Geometry: final body of the model. Coordinates: model frame, mm. Coordinates: 2 decimals unless noted, no trailing zeros. Order: outer loops, then holes, each group sorted by start corner. A loop starts at its lowest first (then second) coordinate and runs counter-clockwise, first axis right, second up. Notation, with made-up numbers: (9, -6.5) -> (28, -6.5) arc R32 ccw to (28, 24.5) -> close; hole circle Ø6 at (-38.75, 4). An arc over 180 degrees is marked (long way). Use one line per item in the form item = value.
Autodesk Fusion 360 part; units mm, degrees
sketch "Sketch1" plane through (0, 0, 0) normal (0, 0, 1) x (1, 0, 0)
  line L0 (0, 0) -> (50, 0)
  line L1 (50, 0) -> (50, 50)
  line L2 (50, 50) -> (0, 50)
  line L3 (0, 50) -> (0, 0)
  line L4 (25, 59.9444) -> (25, -10) construction
  line L5 (-9.9209, 25) -> (60, 25) construction
  line L6 (23.4218, 51.9444) -> (26.5218, 51.9444)
  line L7 (26.5218, 51.9444) -> (26.5218, 25)
  line L8 (26.5218, 25) -> (23.4218, 25)
  line L9 (23.4218, 25) -> (23.4218, 51.9444)
  dimension "d4" = 3.1
extrude "Extrude1" add sketch "Sketch1" along normal blind 3.2 contours L0 L1 L2 L3 L7 L8 L9
chamfer "Chamfer1" distance 3 angle 45 2 edges at (26.5218, 50, 1.6) (23.4218, 50, 1.6)
equation "material_thickness = 3.2 mm"
equation "laser_kerf = 0.1 mm"
equation "chamfer_amount = 3 mm"
equation "d4 = material_thickness - laser_kerf"
equation "d5 = material_thickness"
equation "d7 = chamfer_amount"
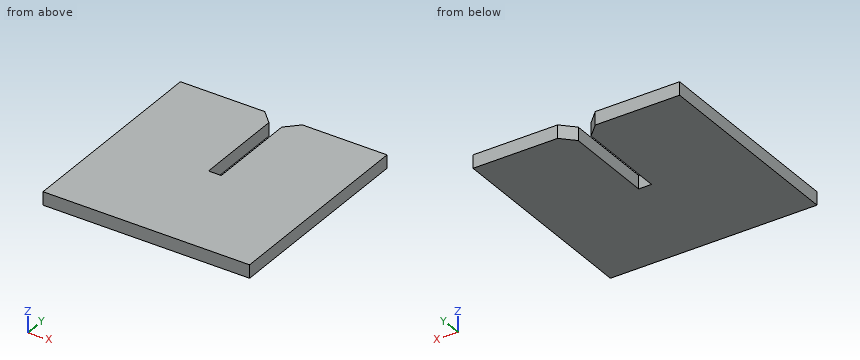
1) Contact query for flat-ended pins moving along their axis: P1, Ø4, axis at x = 16.5, y = 12.5, coming from the -Z side; P2, Ø1.5, axis at x = 25.5, z = 2.5, coming from the +Y side. Output: stop coordinate, or through.
Results found:
P1 = 0
P2 = 25
2) Section B-B, the plane z = 1.4. Output: boundary loops of the cut face in (x, y), and give its area (3 significant figures).
Results found:
outline = (0, 0) -> (50, 0) -> (50, 50) -> (29.52, 50) -> (26.52, 47) -> (26.52, 25) -> (23.42, 25) -> (23.42, 47) -> (20.42, 50) -> (0, 50) -> close
area = 2,410 mm2
3) Section A-A, the plane y = 30. Output: boundary loops of the cut face in (x, z), and give its area (3 significant figures).
Results found:
outline = (0, 0) -> (23.42, 0) -> (23.42, 3.2) -> (0, 3.2) -> close; (26.52, 0) -> (50, 0) -> (50, 3.2) -> (26.52, 3.2) -> close
area = 150 mm2
4) Material intervals for probe 1 along X at (y, z) = (45, 1.2); probe 2 along Y at (x, z) = (24, 1.5); probe 3 along Y at (x, z) = (23, 2.2), sorted ascending. Write a range as from..to.
Results found:
probe_1 = 0..23.42, 26.52..50
probe_2 = 0..25
probe_3 = 0..47.42
